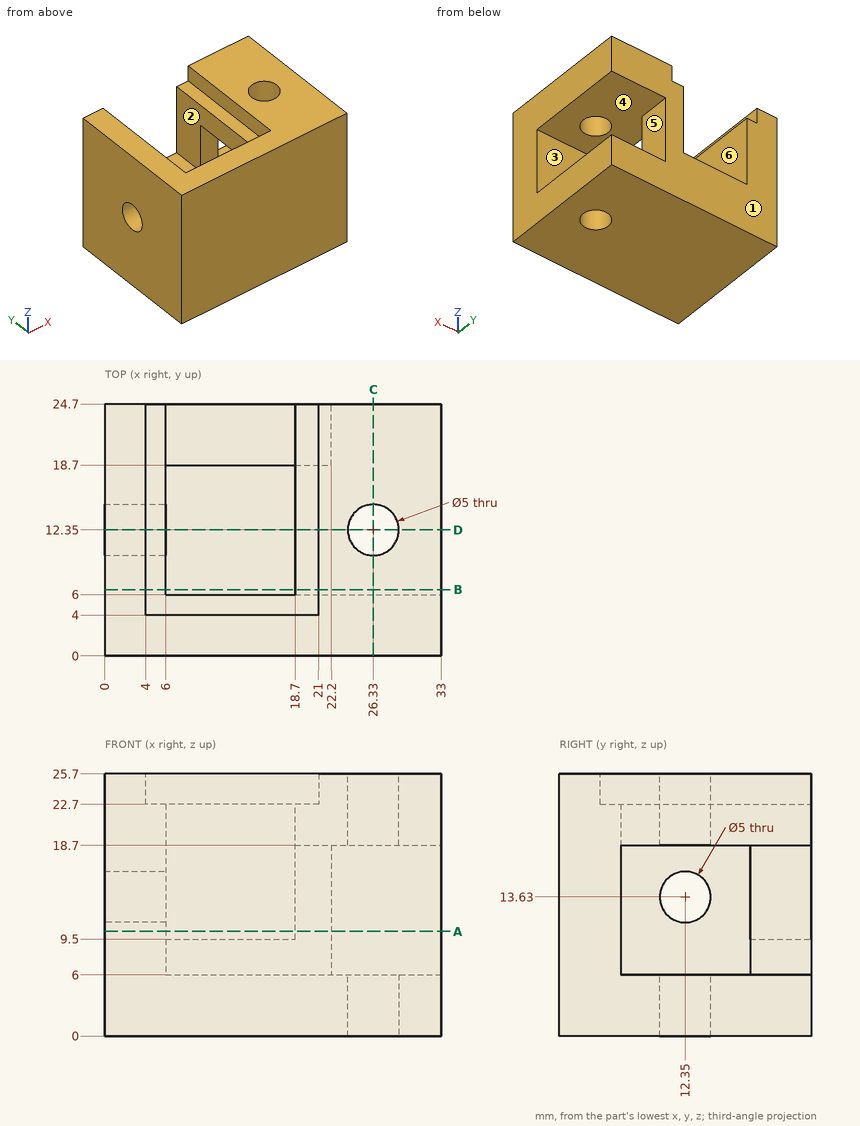
Geometry: see drawing. Coordinates: mm, zero at the bounding-box minimum. A direction names the side the tool comes from. Round coordinates to 2 decimals unless told otherwise and drop trailing zeros. Write each loop counter-clockwise with the first axis right and the second up, starting at its lowest first coordinate (ties: lowest second). Pieces come first, ordered by that corner, then holes. Notation, with made-up numbers: (-19.75, -32.75) - (-8.75, -32.75) arc R16 cw to (-8.75, -6.75) - close; hole circle Ø9 at (-37.5, 45). An arc over 180 degrees is marked (long way). Use CSV: the item, a comma, the result in double quotes. Start each with the question number.
(1) Cut plane A-A, the plane z = 10.25. Return loops of the section in (x, y), and give its area (3 significant figures).
(2) Cut plane C-C, the plane x = 26.33. Return loops of the section in (y, z).
(3) First-contact query: pin 1 Ø3 at (x, y) = (10, 23) entering from +Z; pin 2 Ø3 at (y, z) = (21.5, 9.5) entering from +X; pin 3 Ø8 at (y, z) = (12.35, 13.63) entering from +X. Flat tips, straight axial feed; report the tip coordinate or a pass-through.
(4) Material intervals for probe 1 along Z at (x, y) = (23.5, 20); probe 2 along Y at (x, z) = (26.33, 1.6); probe 3 along X at (y, z) = (8.75, 22.75), sorted ascending. Write a range as [from, to].
(5) Cut plane B-B, the plane y = 6.5. Return loops of the section in (x, z).
(6) Mould query, pull axis Y, two halves, no side actions, for the marked faces 1, 2 and 3. Classes: pulls with the +Y half, pulls with the -Y half, needs draft (parallel to the pull), parting line crosses it, or undercut.
(7) Cut plane D-D, the plane y = 12.35. Return loops of the section in (x, z), and give its area (3 significant figures).
(8) Set-up query: the marked faces 4, 5 and 6. Return all of +Z, -Z, +X, -X, +Y, -Y with unobstructed straight access to the full face (end or side cutting, diameter ignored); none if empty.
Geometry says:
1,outline,"(0, 0) - (33, 0) - (33, 6) - (6, 6) - (6, 24.7) - (0, 24.7) - close; (18.7, 18.7) - (22.2, 18.7) - (22.2, 24.7) - (18.7, 24.7) - close"
1,area,"331 mm²"
2,outline,"(0, 0) - (9.85, 0) - (9.85, 6) - (6, 6) - (6, 18.7) - (9.85, 18.7) - (9.85, 25.7) - (0, 25.7) - close; (14.85, 0) - (24.7, 0) - (24.7, 6) - (14.85, 6) - close; (14.85, 18.7) - (24.7, 18.7) - (24.7, 25.7) - (14.85, 25.7) - close"
3,pin 1,"z = 9.5"
3,pin 2,"x = 22.2"
3,pin 3,"x = 6"
4,probe 1,"[0, 6], [18.7, 25.7]"
4,probe 2,"[0, 9.85], [14.85, 24.7]"
4,probe 3,"[0, 4], [21, 33]"
5,outline,"(0, 0) - (33, 0) - (33, 6) - (6, 6) - (6, 22.7) - (4, 22.7) - (4, 25.7) - (0, 25.7) - close; (18.7, 18.7) - (33, 18.7) - (33, 25.7) - (21, 25.7) - (21, 22.7) - (18.7, 22.7) - close"
6,face 1,"pulls with the +Y half"
6,face 2,"needs draft"
6,face 3,"undercut"
7,outline,"(0, 0) - (23.83, 0) - (23.83, 6) - (6, 6) - (6, 11.13) - (0, 11.13) - close; (0, 16.13) - (6, 16.13) - (6, 22.7) - (4, 22.7) - (4, 25.7) - (0, 25.7) - close; (18.7, 18.7) - (23.83, 18.7) - (23.83, 25.7) - (21, 25.7) - (21, 22.7) - (18.7, 22.7) - close; (28.83, 0) - (33, 0) - (33, 6) - (28.83, 6) - close; (28.83, 18.7) - (33, 18.7) - (33, 25.7) - (28.83, 25.7) - close"
7,area,"308 mm²"
8,face 4,"+X"
8,face 5,"+X, +Y"
8,face 6,"+Z"
